from build123d import *

# Parameters (mm, degrees)
SKETCH1_W            = 135
SKETCH1_H            = 115
BOSS_EXTRUDE1_DEPTH  = 1
SKETCH3_W            = 15
SKETCH3_H            = 15
BOSS_EXTRUDE3_DEPTH  = 1
SKETCH4_W            = 15
SKETCH4_H            = 15
BOSS_EXTRUDE4_DEPTH  = 1
SKETCH5_R            = 1.5
SKETCH5_R_2          = 1.644092979
CUT_EXTRUDE1_DEPTH   = 1
BOSS_EXTRUDE5_START  = -1
SKETCH6_W            = 50
SKETCH6_H            = 15
BOSS_EXTRUDE5_DEPTH  = 1
SKETCH7_W            = 55
SKETCH7_H            = 14.931429571
BOSS_EXTRUDE6_DEPTH  = 1
SKETCH8_W            = 55
SKETCH8_H            = 14.931429571
BOSS_EXTRUDE10_DEPTH = 1
SKETCH9_W            = 50
SKETCH9_H            = 15
BOSS_EXTRUDE11_DEPTH = 1
SKETCH10_W           = 135
SKETCH10_H           = 20
BOSS_EXTRUDE12_DEPTH = 1
SKETCH12_W           = 135
SKETCH12_H           = 20
CUT_EXTRUDE2_DEPTH   = 1
SKETCH14_W           = 51.839856939
SKETCH14_H           = 15
CUT_EXTRUDE3_DEPTH   = 1
SKETCH15_R           = 1.5
CUT_EXTRUDE5_DEPTH   = 10
SKETCH16_R           = 1.5
CUT_EXTRUDE6_DEPTH   = 10
SKETCH17_R           = 1.6
CUT_EXTRUDE9_DEPTH   = 1
SKETCH18_R           = 1.5
SKETCH18_R_2         = 10
CUT_EXTRUDE10_DEPTH  = 10
SKETCH19_R           = 10
CUT_EXTRUDE11_DEPTH  = 10
SKETCH20_W           = 19
SKETCH20_H           = 12
CUT_EXTRUDE12_DEPTH  = 10
SKETCH21_R           = 5
SKETCH21_W           = 1
SKETCH21_H           = 20
CUT_EXTRUDE13_DEPTH  = 10
SKETCH22_R           = 1.5
CUT_EXTRUDE14_DEPTH  = 10
SKETCH23_R           = 1.623611173
SKETCH23_R_2         = 1.5
SKETCH23_R_3         = 1.457682771
SKETCH23_R_4         = 10
SKETCH23_R_5         = 2.633238526
BOSS_EXTRUDE14_DEPTH = 1
SKETCH24_R           = 1.891339509
BOSS_EXTRUDE15_DEPTH = 1
SKETCH25_W           = 2
SKETCH25_H           = 20.001507343
CUT_EXTRUDE15_DEPTH  = 1
SKETCH26_R           = 1.5
CUT_EXTRUDE16_DEPTH  = 1


with BuildPart() as part:
    # Sketch1 → Boss-Extrude1 (new body)
    with BuildSketch(Plane.XY):
        with Locations((-67.5, -57.5)):
            Rectangle(SKETCH1_W, SKETCH1_H)
    extrude(amount=BOSS_EXTRUDE1_DEPTH)

    # Sketch3 → Boss-Extrude3 (add)
    with BuildSketch(Plane(origin=(0, 0, 0), x_dir=(-1, 0, 0), z_dir=(0, 0, -1))):
        with Locations((127.5, -122.5)):
            Rectangle(SKETCH3_W, SKETCH3_H)
        with Locations((127.5, 7.5)):
            Rectangle(SKETCH3_W, SKETCH3_H)
    extrude(amount=-BOSS_EXTRUDE3_DEPTH)

    # Sketch4 → Boss-Extrude4 (add)
    with BuildSketch(Plane(origin=(0, 0, 0), x_dir=(-1, 0, 0), z_dir=(0, 0, -1))):
        with Locations((62.5, -122.5)):
            Rectangle(SKETCH4_W, SKETCH4_H)
        with Locations((62.5, 7.5)):
            Rectangle(SKETCH4_W, SKETCH4_H)
    extrude(amount=-BOSS_EXTRUDE4_DEPTH)

    # Sketch5 → Cut-Extrude1 (cut)
    with BuildSketch(Plane(origin=(0, 0, 0), x_dir=(-1, 0, 0), z_dir=(0, 0, -1))):
        with Locations((62.5, -122.5)):
            Circle(SKETCH5_R)
        with Locations((127.5, -122.5)):
            Circle(SKETCH5_R)
        with Locations((62.5, 7.5)):
            Circle(SKETCH5_R)
        with Locations((127.5, 7.5)):
            Circle(SKETCH5_R_2)
    extrude(amount=-CUT_EXTRUDE1_DEPTH, mode=Mode.SUBTRACT)

    # Sketch6 → Boss-Extrude5 (add)
    with BuildSketch(Plane(origin=(0, 0, 0), x_dir=(-1, 0, 0), z_dir=(0, 0, -1)).offset(BOSS_EXTRUDE5_START)):
        with Locations((95, -122.5)):
            Rectangle(SKETCH6_W, SKETCH6_H)
    extrude(amount=BOSS_EXTRUDE5_DEPTH)

    # Sketch7 → Boss-Extrude6 (add)
    with BuildSketch(Plane(origin=(0, 0, 0), x_dir=(-1, 0, 0), z_dir=(0, 0, -1))):
        with Locations((27.5, -122.465714786)):
            Rectangle(SKETCH7_W, SKETCH7_H)
    extrude(amount=-BOSS_EXTRUDE6_DEPTH)

    # Sketch8 → Boss-Extrude10 (add)
    with BuildSketch(Plane(origin=(0, 0, 0), x_dir=(-1, 0, 0), z_dir=(0, 0, -1))):
        with Locations((27.5, 7.465714786)):
            Rectangle(SKETCH8_W, SKETCH8_H)
    extrude(amount=-BOSS_EXTRUDE10_DEPTH)

    # Sketch9 → Boss-Extrude11 (add)
    with BuildSketch(Plane(origin=(0, 0, 0), x_dir=(-1, 0, 0), z_dir=(0, 0, -1))):
        with Locations((95, 7.5)):
            Rectangle(SKETCH9_W, SKETCH9_H)
    extrude(amount=-BOSS_EXTRUDE11_DEPTH)

    # Sketch10 → Boss-Extrude12 (add)
    with BuildSketch(Plane.XY.offset(1)):
        with Locations((-67.5, 24.931429571)):
            Rectangle(SKETCH10_W, SKETCH10_H)
    extrude(amount=-BOSS_EXTRUDE12_DEPTH)

    # Sketch12 → Cut-Extrude2 (cut)
    with BuildSketch(Plane(origin=(0, 0, 0), x_dir=(-1, 0, 0), z_dir=(0, 0, -1))):
        with Locations((67.5, 24.931429571)):
            Rectangle(SKETCH12_W, SKETCH12_H)
    extrude(amount=-CUT_EXTRUDE2_DEPTH, mode=Mode.SUBTRACT)

    # Sketch14 → Cut-Extrude3 (cut)
    with BuildSketch(Plane(origin=(0, 0, 0), x_dir=(-1, 0, 0), z_dir=(0, 0, -1))):
        with Locations((25.91992847, -122.431429571)):
            Rectangle(SKETCH14_W, SKETCH14_H)
        with Locations((25.91992847, 7.431429571)):
            Rectangle(SKETCH14_W, SKETCH14_H)
    extrude(amount=-CUT_EXTRUDE3_DEPTH, mode=Mode.SUBTRACT)

    # Sketch15 → Cut-Extrude5 (cut)
    with BuildSketch(Plane(origin=(0, 0, 0), x_dir=(-1, 0, 0), z_dir=(0, 0, -1))):
        with Locations((71.839856939, -125)):
            Circle(SKETCH15_R)
        with Locations((113.463350925, -125)):
            Circle(SKETCH15_R)
        with Locations((100, -125)):
            Circle(SKETCH15_R)
        with Locations((87, -125)):
            Circle(SKETCH15_R)
        with Locations((100, 9.931429571)):
            Circle(SKETCH15_R)
        with Locations((87, 9.931429571)):
            Circle(SKETCH15_R)
        with Locations((32.99653198, -109.931429571)):
            Circle(SKETCH15_R)
        with Locations((20, -109.631168863)):
            Circle(SKETCH15_R)
        with Locations((32.99653198, -5.068570429)):
            Circle(SKETCH15_R)
        with Locations((20, -5.068570429)):
            Circle(SKETCH15_R)
    extrude(amount=-CUT_EXTRUDE5_DEPTH, mode=Mode.SUBTRACT)

    # Sketch16 → Cut-Extrude6 (cut)
    with BuildSketch(Plane(origin=(0, 0, 0), x_dir=(-1, 0, 0), z_dir=(0, 0, -1))):
        with Locations((130, -95)):
            Circle(SKETCH16_R)
        with Locations((130, -82)):
            Circle(SKETCH16_R)
        with Locations((130, -33.068570429)):
            Circle(SKETCH16_R)
        with Locations((130, -20.068570429)):
            Circle(SKETCH16_R)
    extrude(amount=-CUT_EXTRUDE6_DEPTH, mode=Mode.SUBTRACT)

    # Sketch17 → Cut-Extrude9 (cut)
    with BuildSketch(Plane(origin=(0, 0, 0), x_dir=(-1, 0, 0), z_dir=(0, 0, -1))):
        with Locations((35, -75.801429571)):
            Circle(SKETCH17_R)
        with Locations((35, -39.201429571)):
            Circle(SKETCH17_R)
        with Locations((71.6, -39.201429571)):
            Circle(SKETCH17_R)
        with Locations((71.6, -75.801429571)):
            Circle(SKETCH17_R)
    extrude(amount=-CUT_EXTRUDE9_DEPTH, mode=Mode.SUBTRACT)

    # Sketch18 → Cut-Extrude10 (cut)
    with BuildSketch(Plane(origin=(0, 0, 0), x_dir=(-1, 0, 0), z_dir=(0, 0, -1))):
        with Locations((115, -20.268570429)):
            Circle(SKETCH18_R)
        with Locations((115, -94.8)):
            Circle(SKETCH18_R)
        with Locations((84, -20.268570429)):
            Circle(SKETCH18_R)
        with Locations((84, -94.8)):
            Circle(SKETCH18_R)
        with Locations((95, -107.048943692)):
            Circle(SKETCH18_R_2)
    extrude(amount=-CUT_EXTRUDE10_DEPTH, mode=Mode.SUBTRACT)

    # Sketch19 → Cut-Extrude11 (cut)
    with BuildSketch(Plane(origin=(0, 0, 0), x_dir=(-1, 0, 0), z_dir=(0, 0, -1))):
        with Locations((94, -7.048943692)):
            Circle(SKETCH19_R)
    extrude(amount=-CUT_EXTRUDE11_DEPTH, mode=Mode.SUBTRACT)

    # Sketch20 → Cut-Extrude12 (cut)
    with BuildSketch(Plane(origin=(0, 0, 0), x_dir=(-1, 0, 0), z_dir=(0, 0, -1))):
        with Locations((119.399363066, -6)):
            Rectangle(SKETCH20_W, SKETCH20_H)
    extrude(amount=-CUT_EXTRUDE12_DEPTH, mode=Mode.SUBTRACT)

    # Sketch21 → Cut-Extrude13 (cut)
    with BuildSketch(Plane(origin=(0, 0, 0), x_dir=(-1, 0, 0), z_dir=(0, 0, -1))):
        with Locations((25.335439778, -57.496285719)):
            Circle(SKETCH21_R)
        with Locations((15.5, -57.498570429)):
            Rectangle(SKETCH21_W, SKETCH21_H)
    extrude(amount=-CUT_EXTRUDE13_DEPTH, mode=Mode.SUBTRACT)

    # Sketch22 → Cut-Extrude14 (cut)
    with BuildSketch(Plane(origin=(0, 0, 0), x_dir=(-1, 0, 0), z_dir=(0, 0, -1))):
        with Locations((53, -20.268570429)):
            Circle(SKETCH22_R)
        with Locations((53, -94.8)):
            Circle(SKETCH22_R)
    extrude(amount=-CUT_EXTRUDE14_DEPTH, mode=Mode.SUBTRACT)

    # Sketch23 → Boss-Extrude14 (add)
    with BuildSketch(Plane(origin=(0, 0, 0), x_dir=(-1, 0, 0), z_dir=(0, 0, -1))):
        with Locations((19.911217807, -5.154578825)):
            Circle(SKETCH23_R)
        with Locations((32.99653198, -5.068570429)):
            Circle(SKETCH23_R_2)
        with Locations((100, 9.931429571)):
            Circle(SKETCH23_R_2)
        with Locations((86.957682771, 9.931429571)):
            Circle(SKETCH23_R_3)
        with Locations((95, -107.048943692)):
            Circle(SKETCH23_R_4)
        with Locations((20, -109.631168863)):
            Circle(SKETCH23_R_2)
        with Locations((32.99653198, -109.931429571)):
            Circle(SKETCH23_R_2)
        with Locations((87, -125)):
            Circle(SKETCH23_R_2)
        with Locations((71.839856939, -125)):
            Circle(SKETCH23_R_5)
        with Locations((100, -125)):
            Circle(SKETCH23_R_2)
        with Locations((113.463350925, -125)):
            Circle(SKETCH23_R_2)
        with Locations((130, -20.068570429)):
            Circle(SKETCH23_R_2)
        with Locations((130, -33.068570429)):
            Circle(SKETCH23_R_2)
        with Locations((130, -82)):
            Circle(SKETCH23_R_2)
        with Locations((130, -95)):
            Circle(SKETCH23_R_2)
        with Locations((115, -20.268570429)):
            Circle(SKETCH23_R_2)
        with Locations((115, -94.8)):
            Circle(SKETCH23_R_2)
    extrude(amount=-BOSS_EXTRUDE14_DEPTH)

    # Sketch24 → Boss-Extrude15 (add)
    with BuildSketch(Plane(origin=(0, 0, 0), x_dir=(-1, 0, 0), z_dir=(0, 0, -1))):
        with Locations((86.989397584, 9.821400511)):
            Circle(SKETCH24_R)
    extrude(amount=-BOSS_EXTRUDE15_DEPTH)

    # Sketch25 → Cut-Extrude15 (cut)
    with BuildSketch(Plane(origin=(0, 0, 0), x_dir=(-1, 0, 0), z_dir=(0, 0, -1))):
        with Locations((14, -57.497816758)):
            Rectangle(SKETCH25_W, SKETCH25_H)
    extrude(amount=-CUT_EXTRUDE15_DEPTH, mode=Mode.SUBTRACT)

    # Sketch26 → Cut-Extrude16 (cut)
    with BuildSketch(Plane(origin=(0, 0, 0), x_dir=(-1, 0, 0), z_dir=(0, 0, -1))):
        with Locations((103, 7.431429571)):
            Circle(SKETCH26_R)
        with Locations((95, 7.431429571)):
            Circle(SKETCH26_R)
        with Locations((87, 7.431429571)):
            Circle(SKETCH26_R)
        with Locations((103, -122.5)):
            Circle(SKETCH26_R)
        with Locations((95, -122.5)):
            Circle(SKETCH26_R)
        with Locations((87, -122.5)):
            Circle(SKETCH26_R)
    extrude(amount=-CUT_EXTRUDE16_DEPTH, mode=Mode.SUBTRACT)


solid = part.part
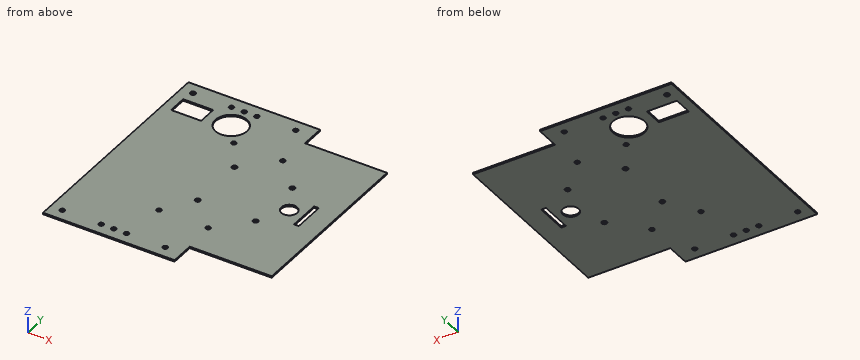
Could you check a few things on this model? Use its own coordinates, in mm. Coordinates: 2 decimals unless noted, no trailing zeros. Order: outer loops, then holes, each group sorted by start corner. A loop starts at its lowest first (then second) coordinate and runs counter-clockwise, first axis right, second up. Notation, with made-up numbers: (14, -24.5) -> (20, -24.5) arc R20 cw to (20, 4.5) -> close; hole circle Ø9 at (71, 60). An arc over 180 degrees is marked (long way). One line per question, with ' | ' between items.
Q1. Imagine slicing it at D-D on z = 0.5. State how many separate pieces and enclosed holes the cut face has, and give its area (3 significant figures).
Return value:
separate pieces: 1 | enclosed holes: 22 | area: 17,200 mm²
Q2. Imagine slicing it at C-C on y = -5. Please give me the cut outline in (x, z).
Return value:
outline: (-135, 0) -> (-128.9, 0) -> (-128.9, 1) -> (-135, 1) -> close; (-109.9, 0) -> (-103.79, 0) -> (-103.79, 1) -> (-109.9, 1) -> close; (-84.21, 0) -> (0, 0) -> (0, 1) -> (-84.21, 1) -> close
Q3. If I drill on L1, parallel to Y at x = -53, z = 0.3; L2, parallel to X at y = -122.5, z = 0.55; L3, parallel to Y at x = -127.5, z = 0.45, over which ranges is the centre line in solid material (lowest first)?
Return value:
L1: -129.93 to -96.3, -93.3 to -21.77, -18.77 to 14.93 | L2: -135 to -129, -126 to -104.5, -101.5 to -96.5, -93.5 to -88.5, -85.5 to -64, -61 to -51.84 | L3: -130 to -124, -121 to -12, 0 to 5.86, 9.14 to 14.93
Q4. Imagine slicing it at B-B on x = -35. Please give me the cut outline in (y, z).
Return value:
outline: (-114.93, 0) -> (-77.4, 0) -> (-77.4, 1) -> (-114.93, 1) -> close; (-74.2, 0) -> (-40.8, 0) -> (-40.8, 1) -> (-74.2, 1) -> close; (-37.6, 0) -> (-0.07, 0) -> (-0.07, 1) -> (-37.6, 1) -> close
Q5. Imagine slicing it at A-A on x = -113. Please give me the cut outline in (y, z).
Return value:
outline: (-130, 0) -> (-12, 0) -> (-12, 1) -> (-130, 1) -> close; (0, 0) -> (14.93, 0) -> (14.93, 1) -> (0, 1) -> close
